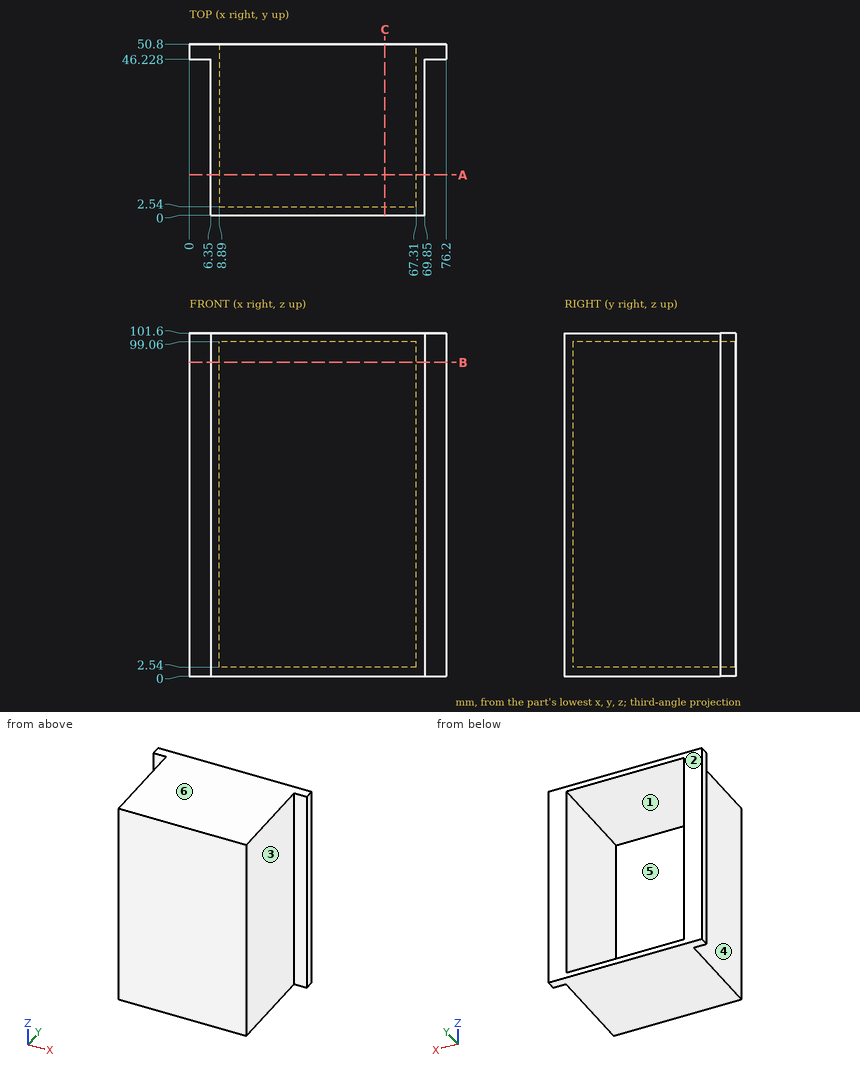
Part print with two shaded views. Sizes in mm from the minimum x, y, z corner. A direction names the side the tool comes from. Round coordinates to 2 decimals unless told otherwise and drop trailing zeros. Loops run counter-clockwise (first coordinate to the right, second up) from the corner with the lowest first, then second, coordinate; pieces in that order, holes last.
Item 1: Pin check, flat tips, straight feed: P1, Ø14.5, axis at y = 23, z = 29.5, coming from the +X side; P2, Ø5, axis at x = 73, z = 35.5, coming from the -Y side; P3, Ø12, axis at y = 37, z = 66.5, coming from the -X side. Stop position of each tip, or through.
Item 2: Drill centre lines: line 1 along X through (y, z) = (37.5, 19); line 2 along Z through (x, y) = (17.5, 42); line 3 along X through (y, z) = (49, 54). Where is each one in solid material? Low to high.
Item 3: Saw through at C-C (x = 58). List the corners of the cut face in (y, z).
Item 4: Which spindle directions (+Z, -Z, +X, -X, +Y, -Y) get a long thin tool onto all of the face, cutting with end or side? Do the marked faces 1, 2 and 3. Say none if no direction does.
Item 5: Two-plate mould, pull along X, no slides. Class the marked faces 4, 5 and 6: released by +X, released by -X, zero draft, split by the parting line, or undercut.
Item 6: Saw through at B-B (z = 93). List the corners of the cut face in (x, y).
Item 7: Saw through at A-A (y = 12). List the corners of the cut face in (x, z), then the cut area to 3 significant figures.
Worked answers:
1. P1: stops at x = 69.85
1. P2: stops at y = 46.23
1. P3: stops at x = 6.35
2. line 1: x = 6.35 to 8.89, 67.31 to 69.85
2. line 2: z = 0 to 2.54, 99.06 to 101.6
2. line 3: x = 0 to 8.89, 67.31 to 76.2
3. outline: (0, 0) - (50.8, 0) - (50.8, 2.54) - (2.54, 2.54) - (2.54, 99.06) - (50.8, 99.06) - (50.8, 101.6) - (0, 101.6) - close
4. face 1: +Y
4. face 2: +Z, -Z, +X, -X, +Y
4. face 3: +Z, -Z, +X, -Y
5. face 4: released by -X
5. face 5: undercut
5. face 6: zero draft
6. outline: (0, 46.23) - (6.35, 46.23) - (6.35, 0) - (69.85, 0) - (69.85, 46.23) - (76.2, 46.23) - (76.2, 50.8) - (67.31, 50.8) - (67.31, 2.54) - (8.89, 2.54) - (8.89, 50.8) - (0, 50.8) - close
7. outline: (6.35, 0) - (69.85, 0) - (69.85, 101.6) - (6.35, 101.6) - close; hole (8.89, 2.54) - (67.31, 2.54) - (67.31, 99.06) - (8.89, 99.06) - close
7. area: 813 mm2
